```python
from build123d import *

# Parameters (mm, degrees)
F0_W     = 95.7072004676
F0_H     = 63.0935970694
F0_R     = 10.9823224345
F0_R_2   = 10.6777928839
F1_DEPTH = 16.51
F2_W     = 63.0935970694
F2_H     = 25.4507996142
F3_DEPTH = 25.4
F4_W     = 65.6336008847
F4_H     = 63.0935970694
F5_DEPTH = 13.208
F6_W     = 14.4779980183
F6_H     = 14.1224008852
F6_W_2   = 13.5636003688
F6_H_2   = 14.4272004122
F7_DEPTH = 23.368


with BuildPart() as f1:
    # F0 (on Top) → F1 (new body)
    with BuildSketch(Plane.XY):
        with Locations((-7.6199993491, 4.5719994232)):
            Rectangle(F0_W, F0_H)
        with Locations((-35.3568010032, 4.5719994232)):
            Circle(F0_R, mode=Mode.SUBTRACT)
        with Locations((13.7159992009, 4.5719994232)):
            Circle(F0_R_2, mode=Mode.SUBTRACT)
    extrude(amount=F1_DEPTH)

    # F2 (on face) → F3 (join)
    with BuildSketch(Plane.YZ.offset(40.2336008847)):
        with Locations((4.5719994232, 12.7253998071)):
            Rectangle(F2_W, F2_H)
    extrude(amount=F3_DEPTH)

    # F4 (on face) → F5 (join)
    with BuildSketch(Plane(origin=(0, 0, 0), x_dir=(1, 0, 0), z_dir=(0, 0, -1))):
        with Locations((32.8168004423, -4.5719994232)):
            Rectangle(F4_W, F4_H)
    extrude(amount=F5_DEPTH)

    # F6 (on face) → F7 (join)
    with BuildSketch(Plane(origin=(-55.4735995829, 0, 0), x_dir=(0, -1, 0), z_dir=(-1, 0, 0))):
        with Locations((-28.8797989488, 23.5712004426)):
            Rectangle(F6_W, F6_H)
        Polygon((-21.6407999396, 16.51), (-36.1187979579, 16.51), (-36.1187979579, 0), (26.9747991115, 0), (26.9747991115, 16.51), (13.4111987427, 16.51), align=None)
        with Locations((20.1929989271, 23.7236002061)):
            Rectangle(F6_W_2, F6_H_2)
    extrude(amount=F7_DEPTH)


solid = f1.part
```
Source: CAD feature listing. Evaluate the final solid. Frame: model axes, mm. A direction names the side the tool comes from. Give positions to 0.01 mm unless a question says otherwise; leave off trailing zeros. Loops run counter-clockwise (first coordinate to the right, second up) from the corner with the lowest first, then second, coordinate; pieces in that order, holes last. Notation, with made-up numbers: (68.25, 23.5) - (103.25, 23.5) arc R29 cw to (103.25, 56.5) - close; hole circle Ø6 at (-39.5, 45.5). An arc over 180 degrees is marked (long way). Use CSV: the item, a comma, the result in double quotes.
1) Line query: line 1 (Y direction, x = -35.5, z = 13); line 2 (Z direction, x = 43, y = 31.5); line 3 (Z direction, x = -64, y = -4). Output: solid intervals per line, ascending.
Worked out:
line 1,"y = -26.97 to -6.41, 15.55 to 36.12"
line 2,"z = -13.21 to 25.45"
line 3,"z = 0 to 16.51"
2) Cut plane C-C (y = -9.5). Output: boundary loops of the cut face in (x, z).
Worked out:
outline,"(-78.84, 0) - (0, 0) - (0, -13.21) - (65.63, -13.21) - (65.63, 25.45) - (40.23, 25.45) - (40.23, 16.51) - (-78.84, 16.51) - close"
3) Mould query, pull axis Y, two halves, no side actions, for faces 1 (the cylindrical face through (23.58, 0.48, 8.14)), 2 (the flat face through (53, 4, 25.451)), 3 (the flat face through (10, -26.975, 9)). Classes: +Y half, -Y half, draft (parallel to the pull), parting line (faces both ways), or undercut.
Worked out:
face 1,"undercut"
face 2,"draft"
face 3,"-Y half"
4) Pin query (flat end, axial travel): P1, Ø10.5, axis at y = 2.5, z = -5.5, coming from the -X side; P2, Ø12, axis at x = -64, y = 23.5, coming from the -Z side; P3, Ø16, axis at x = -62, y = 30.5, coming from the +Z side; P4, Ø8, axis at y = 2.5, z = 25.5, coming from the +X side. Return the tip coordinate at first contact, or that it passes through.
Worked out:
P1,"stops at x = 0"
P2,"stops at z = 0"
P3,"stops at z = 30.63"
P4,"stops at x = 65.63"
5) Set-up query: faces 4 (the flat face through (0, 5, -7)), 5 (the flat face through (-67, 21.641, 23)), 6 (the flat face through (-55.474, -20, 24)). Return all of +Z, -Z, +X, -X, +Y, -Y with unobstructed straight access to the full face (end or side cutting, diameter ignored); none if empty.
Worked out:
face 4,"-Z, -X, +Y, -Y"
face 5,"+Z, -X"
face 6,"+Z, +Y, -Y"
6) Cut plane D-D (y = -3). Output: boundary loops of the cut face in (x, z), and give its area (3 significant figures).
Worked out:
outline,"(-78.84, 0) - (-43.31, 0) - (-43.31, 16.51) - (-78.84, 16.51) - close; (-27.4, 0) - (0, 0) - (0, -13.21) - (65.63, -13.21) - (65.63, 25.45) - (40.23, 25.45) - (40.23, 16.51) - (21.24, 16.51) - (21.24, 0) - (6.19, 0) - (6.19, 16.51) - (-27.4, 16.51) - close"
area,"2,970 mm^2"
7) Cut plane A-A (z = 20). Output: boundary loops of the cut face in (x, y).
Worked out:
outline,"(-78.84, -26.97) - (-55.47, -26.97) - (-55.47, -13.41) - (-78.84, -13.41) - close; (-78.84, 21.64) - (-55.47, 21.64) - (-55.47, 36.12) - (-78.84, 36.12) - close; (40.23, -26.97) - (65.63, -26.97) - (65.63, 36.12) - (40.23, 36.12) - close"
8) Cut plane B-B (x = -39.5). Output: boundary loops of the cut face in (y, z).
Worked out:
outline,"(-26.97, 0) - (-5.6, 0) - (-5.6, 16.51) - (-26.97, 16.51) - close; (14.74, 0) - (36.12, 0) - (36.12, 16.51) - (14.74, 16.51) - close"
